Part model, mm, in its own coordinate system. Face numbers are marked on the shaded views. A direction names the side the tool comes from. Coordinates: 2 decimals unless noted, no trailing zeros. Loops run counter-clockwise (first coordinate to the right, second up) from the corner with the lowest first, then second, coordinate; pieces in that order, holes last. Notation, with made-up numbers: (79, -31) -> (122, -31) arc R23 ccw to (122, -22) -> close; hole circle Ø9 at (-38.5, 17.5). An arc over 180 degrees is marked (long way). One line per question, with ' | ' between items. Start each with the question number.
1) Cut at C-C (y = 1.5). List the corners of the cut face in (x, z), plus the area to 3 significant figures.
2) Cut at B-B (x = 9). List the corners of the cut face in (y, z), plus the area to 3 significant figures.
3) Probe L1, parallel to Z at x = 12, y = 11.75; L2, parallel to X at y = 9.25, z = -25; L3, parallel to Z at x = 18.5, y = 4.5. List the from-to ranges inside material, lowest first. Write a range as from..to.
4) Drop flat-ended pins along their axis: pin 1 (7.5 mm diameter, centred on x = -4.5, y = 4.5, fed in from -Z); pin 2 (2 mm diameter, centred on y = 9, z = -52, fed in from -X); pin 3 (7.5 mm diameter, centred on x = -1.5, y = 7.5, fed in from +Z). Give the stop position or say it passes through.
5) Two-plate mould, pull along Z, no slides. Class the marked faces 1, 2 and 3: released by +Z, released by -Z, zero draft, split by the parting line, or undercut.
6) Cut at A-A (y = 7.5). List the corners of the cut face in (x, z), plus the area to 3 significant figures.
7) Cut at D-D (z = -14.5). List the corners of the cut face in (x, y).
8) 3-axis set-ups, long thin cutter, end or side, ignore diameter. For the marked faces 4 and 5: which of +Z, -Z, +X, -X, +Y, -Y reach the whole face in a straight line?
Autodesk Inventor part; units mm, degrees
ref_plane "YZ Plane" through (0, 0, 0) normal (1, 0, 0) x (0, 1, 0)
ref_plane "XZ Plane" through (0, 0, 0) normal (0, 1, 0) x (-1, 0, 0)
ref_plane "XY Plane" through (0, 0, 0) normal (0, 0, 1) x (1, 0, 0)
sketch "Sketch1" plane through (0, 0, 0) normal (0, 1, 0) x (-1, 0, 0)
  line L0 (20.5369, -73.7451) -> (-17.2994, -73.7451)
  line L1 (-14.2617, -77.74) -> (20.7383, -77.74)
  line L2 (20.7383, -77.74) -> (20.5369, -73.7451)
  line L3 (17.5042, 8.2501) -> (-17.003, 8.2501)
  line L4 (-17.2994, 4.2549) -> (17.7006, 4.2549)
  line L5 (17.7006, 4.2549) -> (17.5042, 8.2501)
  line L6 (-23.7994, -71.2451) -> (-23.7994, 1.7549)
  line L7 (-19.7994, 1.7549) -> (-19.7994, -71.2451)
  arc A0 (-17.2994, 4.2549) -> (-19.7994, 1.7549) centre (-17.2994, 1.7549) ccw
  arc A1 (-17.003, 8.2501) -> (-23.7994, 1.7549) centre (-17.2994, 1.7569) ccw
  arc A2 (-19.7994, -71.2451) -> (-17.2994, -73.7451) centre (-17.2994, -71.2451) ccw
  arc A3 (-23.7994, -71.2451) -> (-14.2617, -77.74) centre (-15.5172, -69.3332) ccw
  point P0 (0, 0)
  dimension "d2" = 4
  dimension "d3" = 4
  dimension "d4" = 35
  dimension "d5" = 35
  dimension "d29" = 78
  dimension "d31" = 73
  dimension "d33" = 2.5
  dimension "d34" = 2.5
  dimension "d36" = 2.5
  dimension "d37" = 4
  dimension "d38" = 6.5
  dimension "d39" = 2.5
  dimension "d41" = 8.5
extrude "Extrusion1" add sketch "Sketch1" along normal blind 15
sketch "Sketch2" plane through (-17.5042, 0, 8.2501) normal (0, 0, 1) x (1, 0, 0)
  circle A0 centre (10, 7.5) radius 3.1
  line L0 (0, 15) -> (34.5072, 15)
  line L1 (0, 0) -> (0, 15)
  point P0 (17.5042, 0)
  dimension "d19" = 6.2
  dimension "d20" = 7.5
  dimension "d21" = 10
extrude "Extrusion2" cut sketch "Sketch2" against normal blind 120
sketch "Sketch3" plane through (12.7652, 0, -83.1298) normal (-1, 0, 0) x (0, 0, 1)
  circle A0 centre (45, 7.5) radius 3.1
  line L0 (0, 15) -> (90, 15)
  line L1 (-6.5, 0) -> (-6.5, 15)
  point P0 (83.1298, 0)
  dimension "d24" = 6.2
  dimension "d25" = 7.5
  dimension "d26" = 51.5
extrude "Extrusion3" [suppressed]
properties part number "Side bar holding bracket"
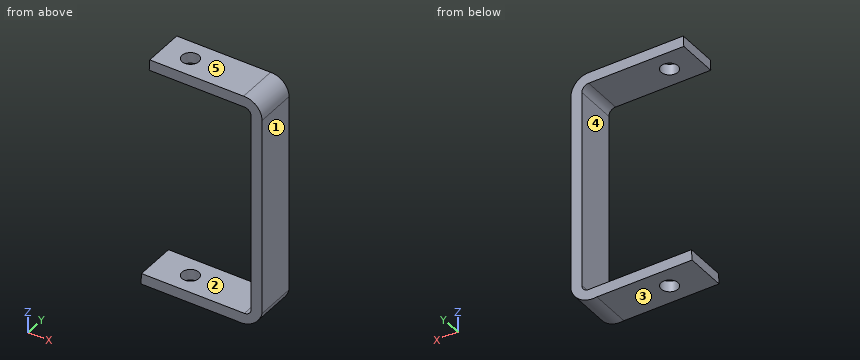
Reported:
1) outline: (-20.74, -77.74) -> (14.26, -77.74) arc R8.5 ccw to (23.8, -71.25) -> (23.8, 1.75) arc R6.5 ccw to (17, 8.25) -> (-17.5, 8.25) -> (-17.7, 4.25) -> (17.3, 4.25) arc R2.5 cw to (19.8, 1.75) -> (19.8, -71.25) arc R2.5 cw to (17.3, -73.75) -> (-20.54, -73.75) -> close | area: 636 mm²
2) outline: (0, -77.74) -> (15, -77.74) -> (15, -73.75) -> (0, -73.75) -> close; (0, 4.25) -> (15, 4.25) -> (15, 8.25) -> (0, 8.25) -> close | area: 120 mm²
3) L1: z = -77.74..-73.75, 4.25..8.25 | L2: x = 19.8..23.8 | L3: z = -77.29..-73.44, 3.95..8.15
4) pin 1: stops at z = -77.74 | pin 2: stops at x = 19.8 | pin 3: stops at z = 8.25
5) face 1: zero draft | face 2: undercut | face 3: released by -Z
6) outline: (-20.74, -77.74) -> (-10.6, -77.74) -> (-10.6, -73.75) -> (-20.54, -73.75) -> close; (-17.7, 4.25) -> (-10.6, 4.25) -> (-10.6, 8.25) -> (-17.5, 8.25) -> close; (-4.4, -77.74) -> (14.26, -77.74) arc R8.5 ccw to (23.8, -71.25) -> (23.8, 1.75) arc R6.5 ccw to (17, 8.25) -> (-4.4, 8.25) -> (-4.4, 4.25) -> (17.3, 4.25) arc R2.5 cw to (19.8, 1.75) -> (19.8, -71.25) arc R2.5 cw to (17.3, -73.75) -> (-4.4, -73.75) -> close | area: 586 mm²
7) outline: (19.8, 0) -> (23.8, 0) -> (23.8, 15) -> (19.8, 15) -> close
8) face 4: -X, +Y, -Y | face 5: +Z, +X, -X, +Y, -Y
